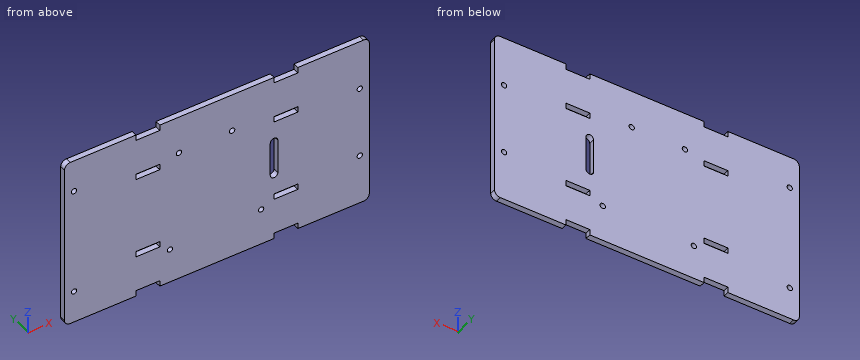
Autodesk Inventor part; units mm, degrees
ref_plane "YZ Plane" through (0, 0, 0) normal (1, 0, 0) x (0, 1, 0)
ref_plane "XZ Plane" through (0, 0, 0) normal (0, 1, 0) x (-1, 0, 0)
ref_plane "XY Plane" through (0, 0, 0) normal (0, 0, 1) x (1, 0, 0)
sketch "Sketch1" plane through (0, 0, 0) normal (0, 1, 0) x (-1, 0, 0)
  line L0 (80, 45) -> (-80, 45)
  line L1 (-80, 45) -> (-80, -45)
  line L2 (-80, -45) -> (80, -45)
  line L3 (80, -45) -> (80, 45)
  line L4 (80, 45) -> (-80, -45) construction
  line L5 (-80, 45) -> (80, -45) construction
  point P0 (0, 0)
  dimension "d0" = 160
  dimension "d1" = 90
extrude "Extrusion1" add sketch "Sketch1" along normal blind 3
sketch "Sketch2" plane through (0, 3, 0) normal (0, 1, 0) x (1, 0, 0)
  line L0 (-42.5, -45) -> (-30, -45)
  line L1 (-30, -45) -> (-30, -41.995)
  line L2 (-30, -41.995) -> (-42.5, -41.995)
  line L3 (-42.5, -41.995) -> (-42.5, -45)
  line L4 (-80, -45) -> (80, -45) construction
  line L5 (0, -45) -> (0, 45) construction
  line L6 (80, 45) -> (-80, 45) construction
  line L7 (-80, 45) -> (-80, -45) construction
  line L8 (-80, 0) -> (80, 0) construction
  line L9 (80, -45) -> (80, 45) construction
  line L10 (-30, -23.095) -> (-42.5, -23.095)
  line L11 (-42.5, -23.095) -> (-42.5, -20.095)
  line L12 (-42.5, -20.095) -> (-30, -20.095)
  line L13 (-30, -20.095) -> (-30, -23.095)
  line L14 (-42.5, 45) -> (-30, 45)
  line L15 (-30, 45) -> (-30, 41.995)
  line L16 (-30, 41.995) -> (-42.5, 41.995)
  line L17 (-42.5, 41.995) -> (-42.5, 45)
  line L18 (-30, 23.095) -> (-42.5, 23.095)
  line L19 (-42.5, 23.095) -> (-42.5, 20.095)
  line L20 (-42.5, 20.095) -> (-30, 20.095)
  line L21 (-30, 20.095) -> (-30, 23.095)
  line L22 (42.5, -45) -> (30, -45)
  line L23 (30, -45) -> (30, -41.995)
  line L24 (30, -41.995) -> (42.5, -41.995)
  line L25 (42.5, -41.995) -> (42.5, -45)
  line L26 (30, -23.095) -> (42.5, -23.095)
  line L27 (42.5, -23.095) -> (42.5, -20.095)
  line L28 (42.5, -20.095) -> (30, -20.095)
  line L29 (30, -20.095) -> (30, -23.095)
  line L30 (30, 45) -> (30, 41.995)
  line L31 (30, 20.095) -> (30, 23.095)
  line L32 (42.5, 45) -> (30, 45)
  line L33 (42.5, 41.995) -> (42.5, 45)
  line L34 (30, 23.095) -> (42.5, 23.095)
  line L35 (42.5, 23.095) -> (42.5, 20.095)
  line L36 (42.5, 20.095) -> (30, 20.095)
  line L37 (30, 41.995) -> (42.5, 41.995)
  point P0 (0, 0)
  point P1 (-36.25, -45)
  point P2 (-36.25, 45)
  point P3 (36.25, -45)
  point P4 (36.25, 45)
  dimension "d4" = 12.5
  dimension "d5" = 3.005
  dimension "d6" = 50
  dimension "d9" = 12.5
  dimension "d10" = 3
  dimension "d11" = 18.9
extrude "Extrusion2" cut sketch "Sketch2" against normal through all
fillet "Fillet1" radius 3 4 edges at (-80, 1.5, 45) (-80, 1.5, -45) (80, 1.5, -45) (80, 1.5, 45)
sketch "Sketch4" plane through (0, 3, 0) normal (0, 1, 0) x (1, 0, 0)
  line L0 (30, 9) -> (30, -9) construction
  line L1 (28, 9) -> (28, -9)
  line L2 (32, -9) -> (32, 9)
  arc A0 (32, 9) -> (28, 9) centre (30, 9) ccw
  arc A1 (28, -9) -> (32, -9) centre (30, -9) ccw
  line L3 (80, -42) -> (80, 42)
  line L4 (42.5, -45) -> (77, -45)
  point P0 (0, 0)
  point P1 (30, 0)
  dimension "d18" = 9
  dimension "d19" = 4
  dimension "d20" = 48
extrude "Extrusion4" cut sketch "Sketch4" against normal through all
sketch "Sketch5" plane through (0, 3, 0) normal (0, 1, 0) x (1, 0, 0)
  circle A0 centre (75, -18.69) radius 1.4
  line L0 (80, -42) -> (80, 42) construction
  line L1 (80, 0) -> (-80, 0) construction
  line L2 (-80, 42) -> (-80, -42) construction
  circle A1 centre (75, 18.69) radius 1.4
  circle A2 centre (-75, 28) radius 1.4
  circle A3 centre (-75, -28) radius 1.4
  circle A4 centre (-19.94, -25) radius 1.4
  circle A5 centre (8, -25) radius 1.4
  line L3 (-30, -45) -> (30, -45) construction
  line L4 (8, -25) -> (23.2, -25) construction
  line L5 (23.2, -25) -> (23.2, 25.8) construction
  circle A6 centre (23.2, 25.8) radius 1.4
  line L6 (-19.94, -25) -> (-24.64, -25) construction
  line L7 (-24.64, -25) -> (-24.64, 26.9) construction
  circle A7 centre (-24.64, 26.9) radius 1.4
  line L8 (-19.94, -25) -> (8, -25) construction
  point P0 (0, 0)
  dimension "d23" = 2.8
  dimension "d24" = 18.69
  dimension "d25" = 5
  dimension "d29" = 2.8
  dimension "d30" = 5
  dimension "d31" = 28
  dimension "d32" = 2.8
  dimension "d33" = 2.8
  dimension "d40" = 15.2
  dimension "d41" = 2.8
  dimension "d43" = 4.7
  dimension "d44" = 2.8
  dimension "d46" = 27.94
  dimension "d47" = 20
  dimension "d48" = 51.9
  dimension "d49" = 50.8
  dimension "d50" = 20
  dimension "d51" = 72
extrude "Extrusion5" cut sketch "Sketch5" against normal through all
properties part number "chassis"
The model under review builds one solid part; all positions refer to its coordinate system, in mm. Give positions to 0.01 mm unless a question says otherwise; leave off trailing zeros. Order: outer loops, then holes, each group sorted by start corner. A loop starts at its lowest first (then second) coordinate and runs counter-clockwise, first axis right, second up. Notation, with made-up numbers: (46, 51) -> (65, 51) arc R24 ccw to (65, 76) -> close; hole circle Ø11 at (8.5, 67.5). An arc over 180 degrees is marked (long way). Write item = value, one per line. Start each with the question number.
(1) Take a section at A-A (x = 37). Write out the cut boundary in (y, z) (3 decimals), plus the area to 3 significant figures.
(2) Take a section at C-C (y = 2.15). State how many separate pieces and enclosed holes the cut face has, plus the area to 3 significant figures.
(3) For L1, parallel to X at y = 0.2, z = -21; L2, parallel to Z at x = 75, y = 0.9; L3, parallel to X at y = 2.3, z = 28, list the stretches that pass through material, from the lowest coordinate up. Write a range as from..to.
(4) Take a section at B-B (z = -3). Write out the cut boundary in (x, y), plus the area to 3 significant figures.
(5) For pin 1 Ø0.9 at (x, y) = (-35.5, 1.5) entering from -Z (3 decimals); pin 2 Ø0.9 at (y, z) = (2, 44) entering from -X; pin 3 Ø1 at (x, z) = (58.5, 32.5) entering from -Y; pin 4 Ø0.9 at (x, y) = (-34.5, 1.5) entering from +Z (3 decimals), all flat-tipped, find the tip position at first contact; note any pin that passes through.
Returned:
q1.outline = (0, -41.995) -> (3, -41.995) -> (3, -23.095) -> (0, -23.095) -> close; (0, -20.095) -> (3, -20.095) -> (3, 20.095) -> (0, 20.095) -> close; (0, 23.095) -> (3, 23.095) -> (3, 41.995) -> (0, 41.995) -> close
q1.area = 234 mm²
q2.separate_pieces = 1
q2.enclosed_holes = 13
q2.area = 14,000 mm²
q3.L1 = -80..-42.5, -30..30, 42.5..80
q3.L2 = -45..-20.09, -17.29..17.29, 20.09..45
q3.L3 = -80..-76.4, -73.6..80
q4.outline = (-80, 0) -> (28, 0) -> (28, 3) -> (-80, 3) -> close; (32, 0) -> (80, 0) -> (80, 3) -> (32, 3) -> close
q4.area = 468 mm²
q5.pin_1 = -41.995
q5.pin_2 = -79.57
q5.pin_3 = 0
q5.pin_4 = 41.995
